Autodesk Inventor part; units mm, degrees
ref_plane "YZ Plane" through (0, 0, 0) normal (1, 0, 0) x (0, 1, 0)
ref_plane "XZ Plane" through (0, 0, 0) normal (0, 1, 0) x (-1, 0, 0)
ref_plane "XY Plane" through (0, 0, 0) normal (0, 0, 1) x (1, 0, 0)
sketch "Boceto1" plane through (0, 0, 0) normal (0, 1, 0) x (-1, 0, 0)
  circle A0 centre (28.5, 0) radius 1.5
  circle A1 centre (28.5, -8) radius 1.5
  circle A2 centre (28.5, 8) radius 1.5
  circle A3 centre (36.5, 0) radius 1.5
  circle A4 centre (20.5, 0) radius 1.5
  circle A5 centre (28.5, 0) radius 47.5
  line L0 (57, 33) -> (43, 33)
  line L1 (43, 33) -> (43, 30)
  line L2 (35.5, 30) -> (35.5, 33)
  line L3 (35.5, 33) -> (21.5, 33)
  line L4 (21.5, 33) -> (21.5, 30)
  line L5 (14, 30) -> (14, 33)
  line L6 (14, 33) -> (0, 33)
  line L7 (43, 30) -> (57, 30)
  line L8 (21.5, 30) -> (35.5, 30)
  line L9 (14, 30) -> (0, 30)
  line L10 (0, 30) -> (0, 33)
  line L11 (57, 33) -> (57, 30)
  line L12 (35.5, -30) -> (35.5, -33)
  line L13 (21.5, -30) -> (35.5, -30)
  line L14 (35.5, -33) -> (21.5, -33)
  line L15 (21.5, -33) -> (21.5, -30)
  line L16 (57, -33) -> (43, -33)
  line L17 (43, -33) -> (43, -30)
  line L18 (43, -30) -> (57, -30)
  line L19 (14, -30) -> (14, -33)
  line L20 (14, -30) -> (0, -30)
  line L21 (14, -33) -> (0, -33)
  line L22 (0, -30) -> (0, -33)
  line L23 (57, -33) -> (57, -30)
extrude "Extrusión1" add sketch "Boceto1" along normal blind 3
sketch "Boceto2" plane through (-28.5, 0, 0) normal (0, -1, 0) x (1, 0, 0)
  circle A0 centre (0, 0) radius 3.5
  point P0 (28.5, 0)
  dimension "d23" = 7
extrude "Extrusión2" cut sketch "Boceto2" against normal blind 10
sketch "Boceto3" plane through (-28.5, 0, 0) normal (0, -1, 0) x (1, 0, 0)
  circle A0 centre (0, 0) radius 4.5
  point P0 (28.5, 0)
  dimension "d26" = 9
extrude "Extrusión3" cut sketch "Boceto3" against normal blind 10
properties part number "base"
Source: CAD feature listing. Evaluate the final solid. Frame: model axes, mm. Round coordinates to 2 decimals unless told otherwise and drop trailing zeros. Loops run counter-clockwise (first coordinate to the right, second up) from the corner with the lowest first, then second, coordinate; pieces in that order, holes last.
Q1. Mould query, pull axis X, two halves, no side actions, for faces 1 (the face through (-28, 0, -10)), 2 (the face through (-35.3, 1.5, 0.9)), 3 (the face through (-35.5, 1, -31)). Classes: pulls with the +X half, pulls with the -X half, needs draft (parallel to the pull), parting line crosses it, or undercut.
Q2. Section A-A, the plane x = -28.5. Return loops of the section in (y, z).
Q3. Section B-B, the plane x = -12. Return loops of the section in (y, z).
Q4. First-contact query: P1, Ø1.5, axis at y = 1.5, z = -31, coming from the +X side; P2, Ø1.5, axis at x = -19.5, y = 1.5, coming from the -Z side; P3, Ø3.5, axis at x = -28.5, z = -8, coming from the +Y side; P4, Ø0.9, axis at x = -4, y = 2, coming from the +Z side. Flat tips, straight axial feed; report the tip coordinate or a pass-through.
Q5. Section C-C, the plane y = 2. State how many separate pieces and enclosed holes the cut face has, plus the area to 3 significant figures.
Q6. Ray query, line 1 (Z direction, x = -28.5, y = 2.15); line 2 (Z direction, x = -46.5, y = 1.85); line 3 (Z direction, x = -32, y = 2.05). Return the intervals inside material, ascending.
Q7. Section D-D, the plane z = -3. Return loops of the section in (x, y).
Solutions:
1. face 1: needs draft
1. face 2: undercut
1. face 3: undercut
2. outline: (0, -47.5) - (3, -47.5) - (3, -33) - (0, -33) - close; (0, -30) - (3, -30) - (3, -9.5) - (0, -9.5) - close; (0, -6.5) - (3, -6.5) - (3, -4.5) - (0, -4.5) - close; (0, 4.5) - (3, 4.5) - (3, 6.5) - (0, 6.5) - close; (0, 9.5) - (3, 9.5) - (3, 30) - (0, 30) - close; (0, 33) - (3, 33) - (3, 47.5) - (0, 47.5) - close
3. outline: (0, -44.54) - (3, -44.54) - (3, -33) - (0, -33) - close; (0, -30) - (3, -30) - (3, 30) - (0, 30) - close; (0, 33) - (3, 33) - (3, 44.54) - (0, 44.54) - close
4. P1: stops at x = 8.12
4. P2: stops at z = -46.78
4. P3: stops at y = 3
4. P4: stops at z = 40.96
5. separate pieces: 1
5. enclosed holes: 11
5. area: 6,740 mm2
6. line 1: z = -47.5 to -33, -30 to -9.5, -6.5 to -4.5, 4.5 to 6.5, 9.5 to 30, 33 to 47.5
6. line 2: z = -43.96 to -33, -30 to 30, 33 to 43.96
6. line 3: z = -47.37 to -33, -30 to -2.83, 2.83 to 30, 33 to 47.37
7. outline: (-75.91, 0) - (-31.85, 0) - (-31.85, 3) - (-75.91, 3) - close; (-25.15, 0) - (18.91, 0) - (18.91, 3) - (-25.15, 3) - close
